Design review of the part built by this model. Coordinates are the model's own, in mm. Round coordinates to 2 decimals unless told otherwise and drop trailing zeros. Order: outer loops, then holes, each group sorted by start corner. A loop starts at its lowest first (then second) coordinate and runs counter-clockwise, first axis right, second up.
from build123d import *

# Parameters (mm, degrees)
F1_DEPTH = 4.7625


with BuildPart() as f1:
    # F0 (on Front) → F1 (new body)
    with BuildSketch(Plane.XZ):
        with BuildLine():
            ThreePointArc((43.350956, 32.385296), (43.963334, 31.69148), (44.562959, 30.986613))
            ThreePointArc((44.562959, 30.986613), (47.902764, 27.518475), (49.119681, 22.86))
            ThreePointArc((49.119681, 22.86), (46.35636, 16.151399), (39.669743, 13.335296))
            Line((39.669743, 13.335296), (128.41962, 13.335296))
            Line((128.41962, 13.335296), (128.41962, 32.385296))
            Line((128.41962, 32.385296), (43.350956, 32.385296))
        make_face()
        with BuildLine():
            ThreePointArc((44.562959, 30.986613), (32.94465, 29.679289), (31.345789, 18.0975))
            ThreePointArc((31.345789, 18.0975), (34.799716, 14.629938), (39.51962, 13.335296))
            Line((39.51962, 13.335296), (39.669743, 13.335296))
            ThreePointArc((39.669743, 13.335296), (46.35636, 16.151399), (49.119681, 22.86))
            ThreePointArc((49.119681, 22.86), (47.902764, 27.518475), (44.562959, 30.986613))
        make_face()
        with BuildLine():
            ThreePointArc((3.302, 36.044068), (19.509924, 30.486733), (31.345789, 18.0975))
            ThreePointArc((31.345789, 18.0975), (32.94465, 29.679289), (44.562959, 30.986613))
            ThreePointArc((44.562959, 30.986613), (43.963334, 31.69148), (43.350956, 32.385296))
            ThreePointArc((43.350956, 32.385296), (23.672268, 45.883291), (0, 48.895))
            Line((0, 48.895), (0, 36.195))
            ThreePointArc((0, 36.195), (1.652724, 36.157247), (3.302, 36.044068))
        make_face()
        with BuildLine():
            ThreePointArc((-3.302, 36.044068), (-1.652724, 36.157247), (0, 36.195))
            Line((0, 36.195), (0, 48.895))
            ThreePointArc((0, 48.895), (-21.386272, 41.429282), (-37.393755, 25.402116))
            Line((-37.393755, 25.402116), (-29.564078, 20.88165))
            ThreePointArc((-29.564078, 20.88165), (-18.0975, 31.345789), (-3.302, 36.044068))
        make_face()
        Polygon((-32.866078, 15.162418), (-37.393755, 25.402116), (-40.695755, 19.682884), align=None)
        with BuildLine():
            ThreePointArc((-32.866078, 15.162418), (-32.139457, 16.647323), (-31.345789, 18.0975))
            ThreePointArc((-31.345789, 18.0975), (-30.486733, 19.509924), (-29.564078, 20.88165))
            Line((-29.564078, 20.88165), (-37.393755, 25.402116))
            Line((-37.393755, 25.402116), (-32.866078, 15.162418))
        make_face()
        with BuildLine():
            Line((-31.345789, 18.0975), (-26.286469, 15.1765))
            Line((-26.286469, 15.1765), (-24.635469, 18.036116))
            Line((-24.635469, 18.036116), (-29.564078, 20.88165))
            ThreePointArc((-29.564078, 20.88165), (-30.486733, 19.509924), (-31.345789, 18.0975))
        make_face()
        with BuildLine():
            Line((-27.937469, 12.316884), (-26.286469, 15.1765))
            Line((-26.286469, 15.1765), (-31.345789, 18.0975))
            ThreePointArc((-31.345789, 18.0975), (-32.139457, 16.647323), (-32.866078, 15.162418))
            Line((-32.866078, 15.162418), (-27.937469, 12.316884))
        make_face()
        with BuildLine():
            Line((0, 30.353), (0, 36.195))
            ThreePointArc((0, 36.195), (-1.652724, 36.157247), (-3.302, 36.044068))
            Line((-3.302, 36.044068), (-3.302, 30.353))
            Line((-3.302, 30.353), (0, 30.353))
        make_face()
        with BuildLine():
            Line((3.302, 30.353), (3.302, 36.044068))
            ThreePointArc((3.302, 36.044068), (1.652724, 36.157247), (0, 36.195))
            Line((0, 36.195), (0, 30.353))
            Line((0, 30.353), (3.302, 30.353))
        make_face()
    extrude(amount=F1_DEPTH)


solid = f1.part
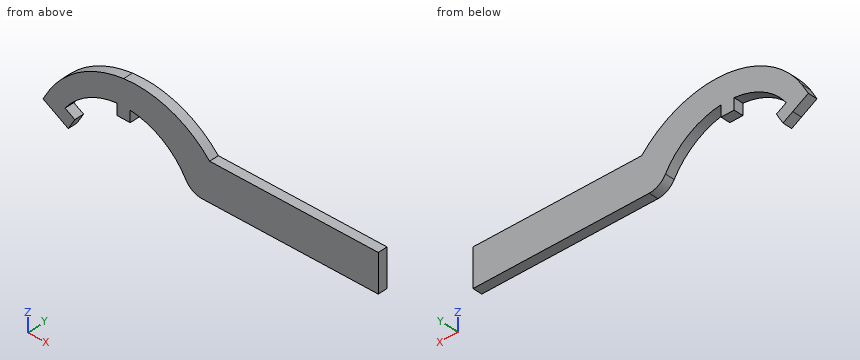
1) To check wall thickness, follow line 1 along X through (y, z) = (-4.2, 31); line 2 along X through (y, z) = (-2.6, 32); line 3 along X through (y, z) = (-0.3, 28). State the ranges of each line that lie inside material, in increasing order.
Results:
line 1: x = -33.33 to -18.68, -3.3 to 3.3, 18.68 to 128.42
line 2: x = -32.47 to -16.91, -3.3 to 3.3, 16.91 to 128.42
line 3: x = -35.65 to -22.94, 22.94 to 128.42
2) Take a section at B-B on z = 27.5. Give the boundary of the cut face in (x, y).
Results:
outline: (-36.01, -4.76) - (-23.53, -4.76) - (-23.53, 0) - (-36.01, 0) - close; (23.53, -4.76) - (128.42, -4.76) - (128.42, 0) - (23.53, 0) - close
3) Take a section at C-C on x = 103. Give the boundary of the cut face in (y, z), plus the area to 3 significant figures.
Results:
outline: (-4.76, 13.34) - (0, 13.34) - (0, 32.39) - (-4.76, 32.39) - close
area: 90.7 mm2
4) Take a section at D-D on z = 47.5. Give the boundary of the cut face in (x, y), plus the area to 3 significant figures.
Results:
outline: (-7.44, -4.76) - (18.66, -4.76) - (18.66, 0) - (-7.44, 0) - close
area: 124 mm2
5) Clearance check with flat-ended pins moving along their axes: P1, Ø2.5, axis at y = -3, z = 33.5, coming from the -X side; P2, Ø1.4, axis at x = 87, y = -1.5, coming from the -Z side. State where each tip first meets the part, or that it passes through.
Results:
P1: stops at x = -32.25
P2: stops at z = 13.34
